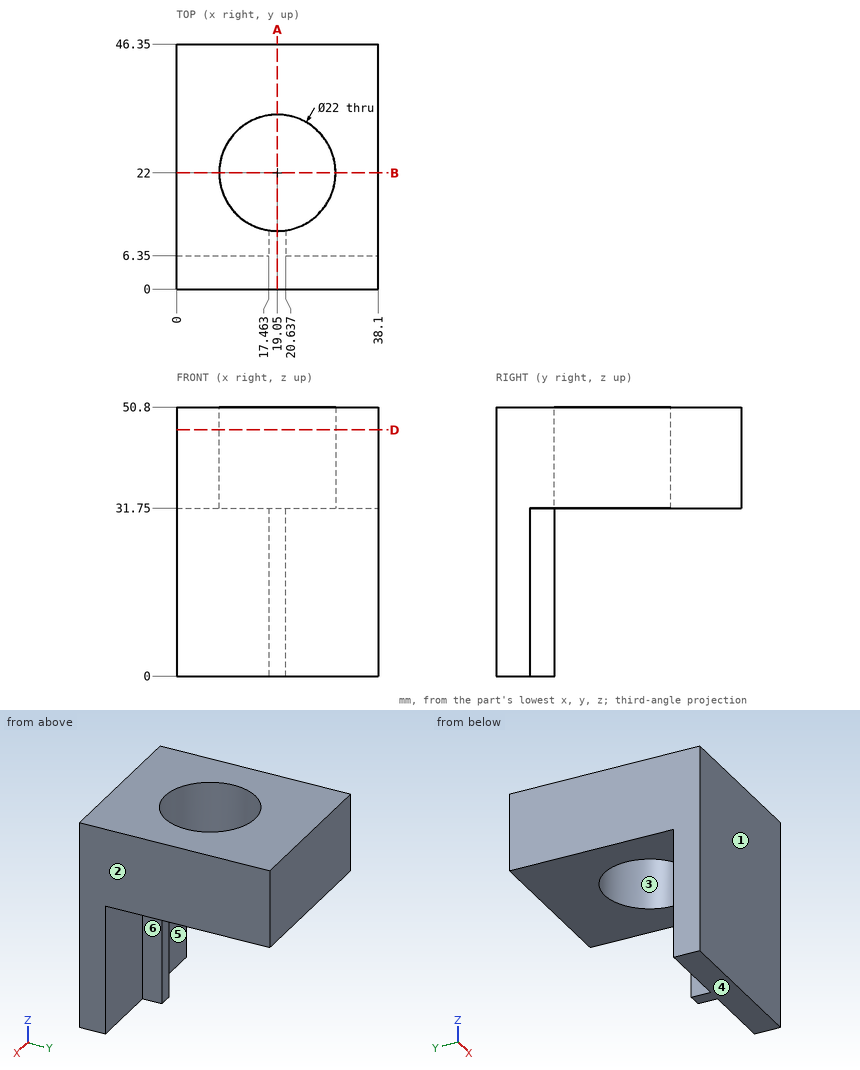
Study the drawing (mm; zero at the part's minimum x, y, z) and answer. A direction names the side the tool comes from. Coordinates: 2 decimals unless noted, no trailing zeros. Write each loop counter-clockwise with the first axis right and the second up, starting at its lowest first coordinate (ties: lowest second). Pieces come first, ordered by that corner, then holes. Notation, with made-up numbers: (89.25, 67) - (131.25, 67) arc R22 cw to (131.25, 93) - close; hole circle Ø10 at (-30, 74.25). An arc over 180 degrees is marked (long way). Answer as a JSON object with one key per item and string values. Group by question number.
1. Consider L1, parallel to Y at x = 19.05, z = 35.5; L2, parallel to X at y = 22, z = 36.5; L3, parallel to Z at x = 2, y = 8.5. Determine where each line is inside the solid, lowest interval first. Write a range as [from, to].
2. A cutting plane is placed at B-B (y = 22). Determine the outline of the cut face in (x, z), plus the area to 3 significant figures.
3. A cutting plane is placed at D-D (z = 46.5). Determine the outline of the cut face in (x, y), plus the area to 3 significant figures.
4. A cutting plane is placed at A-A (x = 19.05). Determine the outline of the cut face in (y, z), plus the area to 3 significant figures.
5. The mould has two halves that part along X. Classify the marked faces 1, 2 and 3: +X half, -X half, draft (parallel to the pull), parting line (faces both ways), or undercut.
6. Each of these flat-tipped pins is pushed along its axis until it touches: P1, Ø14, axis at x = 12, z = 22, coming from the +Y side (1 decimal); P2, Ø11.5, axis at x = 24.5, y = 22.5, coming from the -Z side; P3, Ø1.4, axis at y = 8, z = 21, coming from the -X side; P4, Ø13, axis at x = 19.05, y = 22, coming from the +Z side. Where does it stop, or does it pass through?
7. Which of the six approach directions +Z, -Z, +X, -X, +Y, -Y give full straight-line access (tool end or side, diameter ignored) to the marked faces 4, 5 and 6?
Worked out:
{
 "1": {"L1": "y = [0, 11], [33, 46.35]", "L2": "x = [0, 8.05], [30.05, 38.1]", "L3": "z = [31.75, 50.8]"},
 "2": {"outline": "(0, 31.75) - (8.05, 31.75) - (8.05, 50.8) - (0, 50.8) - close; (30.05, 31.75) - (38.1, 31.75) - (38.1, 50.8) - (30.05, 50.8) - close", "area": "307 mm²"},
 "3": {"outline": "(0, 0) - (38.1, 0) - (38.1, 46.35) - (0, 46.35) - close; hole circle Ø22 at (19.05, 22)", "area": "1,390 mm²"},
 "4": {"outline": "(0, 0) - (11, 0) - (11, 50.8) - (0, 50.8) - close; (33, 31.75) - (46.35, 31.75) - (46.35, 50.8) - (33, 50.8) - close", "area": "813 mm²"},
 "5": {"face 1": "draft", "face 2": "+X half", "face 3": "undercut"},
 "6": {"P1": "stops at y = 11.1", "P2": "stops at z = 31.75", "P3": "stops at x = 17.46", "P4": "passes through"},
 "7": {"face 4": "-Z, +X, -X, +Y, -Y", "face 5": "-Z, -X, +Y", "face 6": "-Z, +X, +Y"}
}
